For this review, use the dimensioned drawing (mm, ordinates from the lowest corner) and the shaded views. A direction names the side the tool comes from. Coordinates: 2 decimals unless noted, no trailing zeros. Loops run counter-clockwise (first coordinate to the right, second up) from the corner with the lowest first, then second, coordinate; pieces in that order, holes last. Notation, with made-up numbers: (39.5, -38) - (77.5, -38) arc R11 cw to (77.5, -20) - close; hole circle Ø6 at (-1, -25). An arc over 180 degrees is marked (long way). Answer in a Markdown table with one row per item. Add a question column.
(1) Machinability: for the marked faces 4 and 5, which of the approach directions +Z, -Z, +X, -X, +Y, -Y give a long, thin tool a straight path to every point of the face, cutting with its end or side? Answer none if there is none.
(2) We need section A-A on x = 15. Write out the cut boundary in (y, z), plus the area to 3 significant figures.
(3) For P1, Ø1.4, axis at x = 12, y = 5, coming from the +Z side; P2, Ø3, axis at x = 13, y = 3, coming from the +Z side; P3, Ø1.5, axis at x = 5, y = 5, coming from the +Z side, all flat-tipped, find the tip position at first contact; note any pin that passes through.
(4) We need section C-C on y = 11. Write out the cut boundary in (x, z).
(5) Mouldability with a two-part tool opening along Y and no side actions: class the marked faces 1, 2 and 3 as +Y half, -Y half, draft (parallel to the pull), parting line (faces both ways), or undercut.
(6) We need section B-B on x = 22. Write out the cut boundary in (y, z).
(7) For line 1 along Y through (x, z) = (22, 4.65); line 2 along Y through (x, z) = (7.5, 6.75); line 3 along Y through (x, z) = (12, 4.85), list the stretches that pass through material, from the lowest coordinate up.
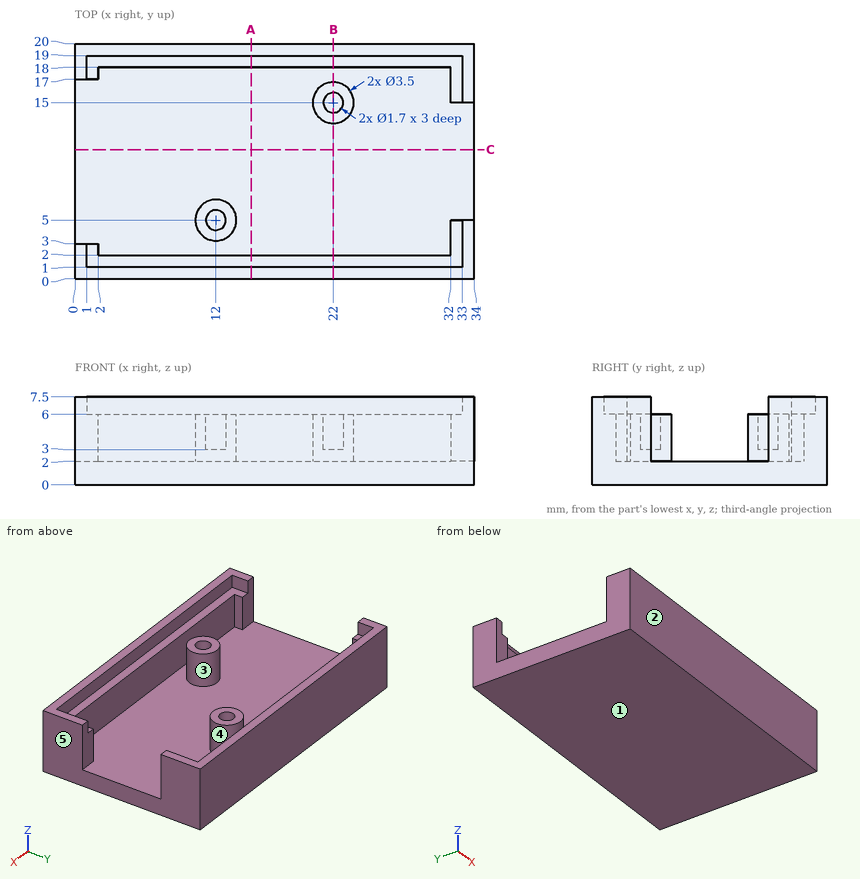
Outcome:
| question | item | result |
|---|---|---|
| 1 | face 4 | +Z |
| 1 | face 5 | +Z, -Z, +X, +Y, -Y |
| 2 | outline | (0, 0) - (20, 0) - (20, 7.5) - (19, 7.5) - (19, 6) - (18, 6) - (18, 2) - (2, 2) - (2, 6) - (1, 6) - (1, 7.5) - (0, 7.5) - close |
| 2 | area | 59.0 mm² |
| 3 | P1 | z = 3 |
| 3 | P2 | z = 6 |
| 3 | P3 | z = 2 |
| 4 | outline | (0, 0) - (34, 0) - (34, 2) - (0, 2) - close |
| 5 | face 1 | draft |
| 5 | face 2 | -Y half |
| 5 | face 3 | undercut |
| 6 | outline | (0, 0) - (20, 0) - (20, 7.5) - (19, 7.5) - (19, 6) - (18, 6) - (18, 2) - (16.75, 2) - (16.75, 6) - (15.85, 6) - (15.85, 3) - (14.15, 3) - (14.15, 6) - (13.25, 6) - (13.25, 2) - (2, 2) - (2, 6) - (1, 6) - (1, 7.5) - (0, 7.5) - close |
| 7 | line 1 | 0 to 2, 13.25 to 14.15, 15.85 to 16.75, 18 to 20 |
| 7 | line 2 | 0 to 1, 19 to 20 |
| 7 | line 3 | 0 to 2, 3.25 to 4.15, 5.85 to 6.75, 18 to 20 |
